Geometry: final body of the model. Coordinates: model frame, mm. Give positions to 0.01 mm unless a question says otherwise; leave off trailing zeros. Write each loop counter-clockwise with the first axis right and the second up, starting at its lowest first coordinate (ties: lowest second). Pieces come first, ordered by that corner, then holes. Notation, with made-up numbers: M 74.5,29 L 117.5,29 A19 ccw 117.5,61 Z; hole C 54,63.5 d8. An arc over 180 degrees is marked long. Answer as a JSON object with one key per item and string values.
from build123d import *

# Parameters (mm, degrees)
ESQUISSE1_R             = 7.7
BOSS_EXTRU_1_DEPTH      = 2.8
ESQUISSE2_R             = 1.9
BOSS_EXTRU_2_DEPTH      = 30
ESQUISSE3_R             = 1.65
ENL_V_MAT_EXTRU_1_DEPTH = 32.91520014
CONG_2_R                = 1


with BuildPart() as part:
    # Esquisse1 → Boss.-Extru.1 (new body)
    with BuildSketch(Plane.XY):
        Circle(ESQUISSE1_R)
    extrude(amount=BOSS_EXTRU_1_DEPTH)

    # Esquisse2 → Boss.-Extru.2 (add)
    with BuildSketch(Plane.XY.offset(2.8)):
        with Locations((0, 4.8)):
            Circle(ESQUISSE2_R)
    extrude(amount=BOSS_EXTRU_2_DEPTH)

    # Esquisse3 → Enlèv. mat.-Extru.1 (cut, through all)
    with BuildSketch(Plane.XY.offset(2.8)):
        Circle(ESQUISSE3_R)
    extrude(amount=-ENL_V_MAT_EXTRU_1_DEPTH, mode=Mode.SUBTRACT)

    # Congé2
    cong_2_edges = [part.edges().sort_by_distance(p)[0] for p in [
        (-1.9, 4.8, 2.8),
    ]]
    fillet(cong_2_edges, radius=CONG_2_R - 0.0001)  # a hair under: the kernel refuses the full size


solid = part.part
1) Line query: line 1 (Y direction, x = 0, z = 0.8); line 2 (Z direction, x = 0.25, y = -7); line 3 (X direction, y = 3.5, z = 11). Output: solid intervals per line, ascending. Write a range as from..to.
Geometry check:
{"line 1": "y = -7.7..-1.65, 1.65..7.7", "line 2": "z = 0..2.8", "line 3": "x = -1.39..1.39"}
2) Cut plane C-C on z = 5. Return loops of the section in (x, y).
Geometry check:
{"outline": "C 0,4.8 d3.8"}
3) Contact query for flat-ended pins moving along their axis: P1, Ø4, axis at x = 4.5, z = 16, coming from the -Y side; P2, Ø6, axis at x = -2, z = 24, coming from the -Y side. Output: stop coordinate, or through.
Geometry check:
{"P1": "passes through", "P2": "stops at y = 2.9"}
4) Cut plane D-D on y = 4.8. Return loops of the section in (x, z), and give its area (3 significant figures).
Geometry check:
{"outline": "M -6.02,0 L 6.02,0 L 6.02,2.8 L 2.9,2.8 A1 cw 1.9,3.8 L 1.9,32.8 L -1.9,32.8 L -1.9,3.8 A1 cw -2.9,2.8 L -6.02,2.8 Z", "area": "148 mm2"}
5) Cut plane A-A on y = 0. Return loops of the section in (x, z).
Geometry check:
{"outline": "M -7.7,0 L -1.65,0 L -1.65,2.8 L -7.7,2.8 Z; M 1.65,0 L 7.7,0 L 7.7,2.8 L 1.65,2.8 Z"}
6) Pull-direction query (Y, two-part tool) for faces 1 (the flat face through (0, 5, 32.8)), 2 (the cylindrical face through (-0.412, 2.945, 18.097)), 3 (the cylindrical face through (-1.216, 1.115, 1.42)); classes: pulls with the +Y half, pulls with the -Y half, needs draft (parallel to the pull), parting line crosses it, or undercut.
Geometry check:
{"face 1": "needs draft", "face 2": "parting line crosses it", "face 3": "undercut"}
